CAD build for the part. Positions are in the model's coordinates, mm. A direction names the side the tool comes from. Give positions to 0.01 mm unless a question says otherwise; leave off trailing zeros. Write each loop counter-clockwise with the first axis right and the second up, starting at its lowest first coordinate (ties: lowest second). Pieces come first, ordered by that corner, then holes. Notation, with made-up numbers: (71, 41) -> (84, 41) arc R10 ccw to (84, 47) -> close; hole circle Ø9 at (27.25, 18). An arc over 180 degrees is marked (long way). Answer as a JSON object with one key per item and string values.
Autodesk Inventor part; units mm, degrees
ref_plane "YZ Plane" through (0, 0, 0) normal (1, 0, 0) x (0, 1, 0)
ref_plane "XZ Plane" through (0, 0, 0) normal (0, 1, 0) x (-1, 0, 0)
ref_plane "XY Plane" through (0, 0, 0) normal (0, 0, 1) x (1, 0, 0)
sketch "Sketch3" plane through (0, 0, 0) normal (0, 1, 0) x (-1, 0, 0)
  line L0 (0, 0) -> (0, -65)
  line L1 (0, -65) -> (25, -65)
  line L2 (25, -65) -> (25, 0)
  line L3 (25, 0) -> (0, 0)
  dimension "d8" = 65
  dimension "d9" = 25
  dimension "d10" = 65
extrude "Extrusion2" add sketch "Sketch3" along normal blind 170
sketch "Sketch4" plane through (0, 0, 0) normal (1, 0, 0) x (0, 0, -1)
  line L0 (65, 170) -> (0, 170)
  line L1 (0, 170) -> (32.5, 170)
  line L2 (65, 0) -> (65, 170)
  line L3 (32.5, 170) -> (32.5, 135)
  circle A0 centre (32.5, 135) radius 23.75
  point P0 (0, 0)
  dimension "d13" = 32.5
  dimension "d15" = 35
  dimension "d16" = 47.5
extrude "Extrusion3" cut sketch "Sketch4" against normal blind 12.5
sketch "Sketch6" plane through (0, 0, 0) normal (1, 0, 0) x (0, 0, -1)
  line L0 (65, 0) -> (0, 0)
  line L1 (0, 0) -> (32.5, 0)
  line L2 (32.5, 0) -> (11.2, 0)
  line L3 (11.2, 0) -> (53.8, 0)
  line L4 (53.8, 0) -> (53.8, 100)
  line L5 (53.8, 100) -> (65, 100)
  line L6 (65, 0) -> (65, 170)
  line L7 (65, 0) -> (53.8, 0)
  line L8 (11.2, 0) -> (0, 0)
  line L9 (0, 0) -> (0, 170)
  line L10 (0, 100) -> (11.2, 100)
  line L11 (11.2, 100) -> (11.2, 0)
  dimension "d23" = 21.3
  dimension "d24" = 42.6
  dimension "d25" = 100
extrude "Extrusion4" add sketch "Sketch6" along normal blind 39.5
sketch "Sketch7" plane through (39.5, 0, 0) normal (1, 0, 0) x (0, 0, -1)
  line L0 (65, 0) -> (0, 0)
  line L1 (53.8, 0) -> (53.8, 100)
  line L2 (65, 0) -> (53.8, 0)
  line L3 (53.8, 0) -> (45.8, 0)
  line L4 (45.8, 0) -> (45.8, 100)
  line L5 (53.8, 100) -> (65, 100)
  line L6 (45.8, 100) -> (65, 100)
  line L7 (65, 0) -> (65, 170)
  line L8 (65, 100) -> (65, 0)
  line L9 (11.2, 100) -> (11.2, 0)
  line L10 (11.2, 0) -> (19.2, 0)
  line L11 (19.2, 0) -> (19.2, 100)
  line L12 (0, 100) -> (11.2, 100)
  line L13 (19.2, 100) -> (0, 100)
  line L14 (0, 100) -> (0, 0)
  dimension "d28" = 8
  dimension "d29" = 8
extrude "Extrusion5" add sketch "Sketch7" along normal blind 8.5
sketch "Sketch8" plane through (48, 0, 0) normal (1, 0, 0) x (0, 0, -1)
  circle A0 centre (32.5, 135) radius 23.75
  circle A1 centre (32.5, 135) radius 76.5
  line L0 (65, 0) -> (0, 0)
  line L1 (32.5, 0) -> (32.5, 58.5)
  line L2 (32.5, 58.5) -> (32.5, 57.9046)
  line L3 (32.5, 58.5) -> (32.5, 40.5)
  circle A2 centre (32.5, 49.5) radius 9
  line L4 (32.5, 49.5) -> (32.5, 28.5)
  line L5 (32.5, 28.5) -> (53.5, 28.5)
  line L6 (53.8, 0) -> (53.8, 100)
  line L7 (53.5, 28.5) -> (53.5, 70.5)
  line L8 (53.5, 70.5) -> (11.5, 70.5)
  line L9 (11.2, 100) -> (11.2, 0)
  line L10 (11.5, 70.5) -> (11.5, 28.5)
  line L11 (11.5, 28.5) -> (32.5, 28.5)
  line L12 (32.5, 28.5) -> (32.5, 16.4931)
  line L13 (32.5, 28.5) -> (32.5, 18.5)
  line L14 (32.5, 18.5) -> (55.5, 18.5)
  line L15 (55.5, 18.5) -> (55.5, 8)
  line L16 (55.5, 8) -> (9.5, 8)
  line L17 (9.5, 8) -> (9.5, 18.5)
  line L18 (9.5, 18.5) -> (32.5, 18.5)
  point P0 (11.2, 18.5)
  point P1 (11.2, 8)
  point P2 (53.8, 8)
  point P3 (53.8, 18.5)
  dimension "d32" = 153
  dimension "d33" = 18
  dimension "d34" = 21
  dimension "d38" = 42
  dimension "d39" = 42
  dimension "d42" = 42
  dimension "d43" = 10
  dimension "d44" = 23
  dimension "d45" = 10.5
  dimension "d46" = 46
  dimension "d47" = 10.5
extrude "Extrusion6" cut sketch "Sketch8" against normal through all contours L18 L1 L16 L9 | L6 L16 L1 L14
sketch "Sketch9" plane through (-12.5, 135, -32.5) normal (1, 0, 0) x (0, 0, -1)
  circle A0 centre (0, 0) radius 12.5
  point P0 (-32.5, -135)
  dimension "d50" = 25
extrude "Extrusion7" cut sketch "Sketch9" against normal through all
sketch "Sketch10" plane through (-25, 0, -65) normal (-1, 0, 0) x (0, 0, 1)
  line L0 (65, 0) -> (45.8, 0)
  line L1 (65, 0) -> (0, 0)
  line L2 (0, 0) -> (0, 170)
  line L3 (0, 170) -> (65, 170)
  line L4 (65, 170) -> (65, 0)
extrude "Extrusion8" cut sketch "Sketch10" against normal blind 7
sketch "Sketch11" plane through (48, 0, 0) normal (1, 0, 0) x (0, 0, -1)
  circle A0 centre (32.5, 135) radius 12.5
  line L0 (32.5, 135) -> (32.5, 18.5)
  line L1 (11.2, 18.5) -> (53.8, 18.5)
  point P0 (0, 0)
sketch "Sketch12" plane through (-12.5, 135, -32.5) normal (1, 0, 0) x (0, 0, -1)
  circle A0 centre (0, 0) radius 12.5
  circle A1 centre (0, 0) radius 14.65
  circle A2 centre (0, 0) radius 21.85
  point P0 (-32.5, -135)
  dimension "d55" = 29.3
  dimension "d56" = 43.7
extrude "Extrusion9" cut sketch "Sketch12" against normal blind 2 contours A2
sketch "Sketch13" plane through (0, 170, 0) normal (1, 0, 0) x (0, 0, -1)
  line L0 (65, -170) -> (65, 0)
  circle A0 centre (32.5, -35) radius 21.85
  line L1 (0, 0) -> (0, -170)
  circle A1 centre (32.5, -35) radius 14.65
  circle A2 centre (32.5, -35) radius 23.75
  line L2 (65, 0) -> (48.6607, -17.5962)
  line L3 (16.3393, -17.5962) -> (0, 0)
  circle A3 centre (56.8304, -8.7981) radius 2.75
  circle A4 centre (8.1696, -8.7981) radius 2.75
  dimension "d59" = 5.5
  dimension "d60" = 5.5
extrude "Extrusion10" cut sketch "Sketch13" against normal through all contours A4 L3 | L3 A4 | A3 L2 | L2 A3
sketch "Sketch14" plane through (0, 0, -11.2) normal (1, 0, 0) x (0, 0, -1)
  line L0 (0, 0) -> (42.6, 0)
  point P0 (-11.2, 0)
sketch "Sketch15" plane through (0, 0, -11.2) normal (1, 0, 0) x (0, 0, -1)
  line L0 (0, 0) -> (0, 8)
  line L1 (0, 0) -> (0, -8)
  line L2 (0, -8) -> (42.6, -8)
  line L3 (34.6, 0) -> (42.6, 0)
  line L4 (42.6, -8) -> (42.6, 0)
  line L5 (42.6, 0) -> (0, 0)
  point P0 (-11.2, 0)
  dimension "d63" = 8
extrude "Extrusion11" add sketch "Sketch15" against normal blind 18
sketch "Sketch16" plane through (0, 8, -11.2) normal (1, 0, 0) x (0, 0, -1)
  line L0 (0, -8) -> (8, -8)
  line L1 (8, -8) -> (12, -8)
  line L2 (42.6, -16) -> (0, -16)
  line L3 (34.6, 0) -> (34.6, -8)
  line L4 (12, -8) -> (34.6, -8)
  line L5 (34.6, -8) -> (29.6, -8)
  circle A0 centre (29.6, -8) radius 2.75
  circle A1 centre (12, -8) radius 2.75
  point P0 (-11.2, -8)
  dimension "d66" = 4
  dimension "d67" = 5
  dimension "d68" = 5.5
  dimension "d69" = 5.5
extrude "Extrusion12" cut sketch "Sketch16" against normal through all
sketch "Sketch17" plane through (0, 170, 0) normal (1, 0, 0) x (0, 0, -1)
  point P0 (0, -170)
sketch "Sketch18" plane through (-18, 0, -65) normal (-1, 0, 0) x (0, 0, 1)
  point P0 (65, 0)
sketch "Sketch19" plane through (-18, 0, -65) normal (-1, 0, 0) x (0, 0, 1)
  point P0 (65, 0)
properties part number "base"
1) Slice it at D-D (z = -23.2). List the corners of the cut face in (x, y).
Model answer:
{"outline": "(-18, -8) -> (0, -8) -> (0, -2.75) -> (-18, -2.75) -> close; (-18, 2.75) -> (0, 2.75) -> (0, 8) -> (-18, 8) -> close; (-18, 18.5) -> (0, 18.5) -> (0, 113.15) -> (-12.5, 113.15) -> (-12.5, 115.23) -> (-14.5, 115.23) -> (-14.5, 123.68) -> (-12.5, 123.68) -> (-12.5, 126.65) -> (-18, 126.65) -> close; (-18, 143.35) -> (-12.5, 143.35) -> (-12.5, 146.32) -> (-14.5, 146.32) -> (-14.5, 154.77) -> (-12.5, 154.77) -> (-12.5, 156.85) -> (0, 156.85) -> (0, 170) -> (-18, 170) -> close"}
2) Slice it at B-B (y = 135). List the corners of the cut face in (x, z).
Model answer:
{"outline": "(-18, -65) -> (0, -65) -> (0, -56.25) -> (-12.5, -56.25) -> (-12.5, -54.35) -> (-14.5, -54.35) -> (-14.5, -47.15) -> (-12.5, -47.15) -> (-12.5, -45) -> (-18, -45) -> close; (-18, -20) -> (-12.5, -20) -> (-12.5, -17.85) -> (-14.5, -17.85) -> (-14.5, -10.65) -> (-12.5, -10.65) -> (-12.5, -8.75) -> (0, -8.75) -> (0, 0) -> (-18, 0) -> close"}
3) Wall check: probe 1 along Y at (x, z) = (-9, -32); probe 2 along Z at (x, y) = (23, 4); probe 3 along Y at (x, z) = (-10, -39). Give the ranges that are in metal, low to high.
Model answer:
{"probe 1": "y = -8 to 8, 18.5 to 111.26, 158.74 to 170", "probe 2": "z = -65 to -53.8, -11.2 to 0", "probe 3": "y = -8 to -2.08, 2.08 to 8, 18.5 to 112.16, 157.84 to 170"}
4) 3-axis set-ups, long thin cutter, end or side, ignore diameter. For faces 1 (the flat face through (39.5, 4, -50)), 2 (the flat face through (44, 59, -19.2)), 3 (the flat face through (0, 93, -32)), 4 (the flat face through (44, 8, -15)), 5 (the cylindrical face through (-13.49, 126.09, -20.87)): which of +Z, -Z, +X, -X, +Y, -Y reach the whole face in a straight line?
Model answer:
{"face 1": "+Y, -Y", "face 2": "+X, +Y, -Y", "face 3": "+Y", "face 4": "+X, -X", "face 5": "+X"}
5) Pin check, flat tips, straight feed: pin 1 (2.5 mm diameter, centred on x = 42, z = -48, fed in from -Y); pin 2 (5 mm diameter, centred on y = 161.2, z = -56.83, fed in from +X); pin 3 (9.5 mm diameter, centred on x = 26.5, z = -59.5, fed in from +Y); pin 4 (8 mm diameter, centred on y = 35, z = -31, fed in from +X). Stop position of each tip, or through.
Model answer:
{"pin 1": "stops at y = 0", "pin 2": "passes through", "pin 3": "stops at y = 100", "pin 4": "stops at x = 0"}
6) Mould opens along Z. For faces 6 (the flat face through (44, 4, -45.8)), 7 (the flat face through (-9, -4, -53.8)), 8 (the flat face through (-9, -4, -11.2)) say: released by +Z, released by -Z, zero draft, split by the parting line, or undercut.
Model answer:
{"face 6": "undercut", "face 7": "released by -Z", "face 8": "released by +Z"}
7) Slice it at A-A (x = 15). List the corners of the cut face in (y, z).
Model answer:
{"outline": "(0, -65) -> (100, -65) -> (100, -53.8) -> (0, -53.8) -> close; (0, -11.2) -> (100, -11.2) -> (100, 0) -> (0, 0) -> close"}
8) Slice it at C-C (z = -32.5). List the corners of the cut face in (x, y).
Model answer:
{"outline": "(-18, -8) -> (0, -8) -> (0, 8) -> (-18, 8) -> close; (-18, 18.5) -> (0, 18.5) -> (0, 111.25) -> (-12.5, 111.25) -> (-12.5, 113.15) -> (-14.5, 113.15) -> (-14.5, 120.35) -> (-12.5, 120.35) -> (-12.5, 122.5) -> (-18, 122.5) -> close; (-18, 147.5) -> (-12.5, 147.5) -> (-12.5, 149.65) -> (-14.5, 149.65) -> (-14.5, 156.85) -> (-12.5, 156.85) -> (-12.5, 158.75) -> (0, 158.75) -> (0, 170) -> (-18, 170) -> close"}
